Source: CAD feature listing. Evaluate the final solid. Frame: model axes, mm. Round coordinates to 2 decimals unless told otherwise and drop trailing zeros.
Item 1: Ray query, L1, parallel to Y at x = -9.5, z = 139; L2, parallel to Y at x = -16.75, z = 102; L3, parallel to Y at x = -3.75, z = 65. Return the intervals inside material, ascending.
Item 2: First-contact query: P1, Ø3, axis at x = -13, z = 129.5, coming from the -Y side; P2, Ø1.8, axis at y = -9, z = 234, coming from the +X side. Flat tips, straight axial feed; report the tip coordinate or a pass-through.
Item 3: Pull-direction query (X, two-part tool) for faces 1 (the flat face through (-2.505, -4, 168)), 2 (the flat face through (-12, -5.11, 172)), 3 (the flat face through (-19, -19.91, 168)); classes: released by +X, released by -X, zero draft, split by the parting line, or undercut.
```python
from build123d import *

# Parameters (mm, degrees)
ESQUISSE1_W             = 20
ESQUISSE1_H             = 20
BOSS_EXTRU_1_DEPTH      = 340
ESQUISSE2_W             = 1.2
ESQUISSE2_H             = 5.5
ESQUISSE2_W_2           = 5.5
ESQUISSE2_H_2           = 1.2
ENL_V_MAT_EXTRU_1_DEPTH = 341
ENL_V_MAT_EXTRU_2_DEPTH = 341
ESQUISSE4_R             = 2.5
ENL_V_MAT_EXTRU_3_DEPTH = 341


with BuildPart() as part:
    # Esquisse1 → Boss.-Extru.1 (new body)
    with BuildSketch(Plane.XY):
        with Locations((-12.505109137, -9.909560068)):
            Rectangle(ESQUISSE1_W, ESQUISSE1_H)
    extrude(amount=BOSS_EXTRU_1_DEPTH)

    # Esquisse2 → Enlèv. mat.-Extru.1 (cut, through all)
    with BuildSketch(Plane.XY.offset(340)):
        with Locations((-21.905109137, -9.909560068)):
            Rectangle(ESQUISSE2_W, ESQUISSE2_H)
        with Locations((-12.505109137, -0.509560068)):
            Rectangle(ESQUISSE2_W_2, ESQUISSE2_H_2)
        with Locations((-3.105109137, -9.909560068)):
            Rectangle(ESQUISSE2_W, ESQUISSE2_H)
        with Locations((-12.505109137, -19.309560068)):
            Rectangle(ESQUISSE2_W_2, ESQUISSE2_H_2)
    extrude(amount=-ENL_V_MAT_EXTRU_1_DEPTH, mode=Mode.SUBTRACT)

    # Esquisse3 → Enlèv. mat.-Extru.2 (cut, through all)
    with BuildSketch(Plane.XY.offset(340)):
        Polygon((-21.305109137, -15.909560068), (-20.305109137, -15.909560068), (-17.305109137, -12.909560068), (-17.305109137, -6.909560068), (-20.305109137, -3.909560068), (-21.305109137, -3.909560068), align=None)
        Polygon((-18.505109137, -1.109560068), (-6.505109137, -1.109560068), (-6.505109137, -2.109560068), (-9.505109137, -5.109560068), (-15.505109137, -5.109560068), (-18.505109137, -2.109560068), align=None)
        Polygon((-3.705109137, -3.909560068), (-4.705109137, -3.909560068), (-7.705109137, -6.909560068), (-7.705109137, -12.909560068), (-4.705109137, -15.909560068), (-3.705109137, -15.909560068), align=None)
        Polygon((-6.505109137, -18.709560068), (-18.505109137, -18.709560068), (-18.505109137, -17.709560068), (-15.505109137, -14.709560068), (-9.505109137, -14.709560068), (-6.505109137, -17.709560068), align=None)
    extrude(amount=-ENL_V_MAT_EXTRU_2_DEPTH, mode=Mode.SUBTRACT)

    # Esquisse4 → Enlèv. mat.-Extru.3 (cut, through all)
    with BuildSketch(Plane.XY.offset(340)):
        with Locations((-12.505109137, -9.909560068)):
            Circle(ESQUISSE4_R)
    extrude(amount=-ENL_V_MAT_EXTRU_3_DEPTH, mode=Mode.SUBTRACT)


solid = part.part
```
Data:
1. L1: y = -19.91 to -18.71, -14.71 to -5.1, -1.11 to 0.09
1. L2: y = -19.91 to -18.71, -15.95 to -3.86, -1.11 to 0.09
1. L3: y = -19.91 to -15.91, -3.91 to 0.09
2. P1: stops at y = -14.71
2. P2: stops at x = -7.71
3. face 1: released by +X
3. face 2: undercut
3. face 3: zero draft
